```python
from build123d import *

# Parameters (mm, degrees)
SKETCH2_R           = 1.55
SKETCH2_R_2         = 6
SKETCH2_R_3         = 2.5
BOSS_EXTRUDE1_DEPTH = 3.2


with BuildPart() as part:
    # Sketch2 → Boss-Extrude1 (new body)
    with BuildSketch(Plane.XY):
        with BuildLine():
            Line((-37.606688888, -62.799107474), (37.606688888, -62.799107474))
            ThreePointArc((37.606688888, -62.799107474), (48.801571995, -62.445486831), (59.972328875, -61.630228563))
            ThreePointArc((59.972328875, -61.630228563), (73.015089975, -59.821162533), (85.558909279, -55.816298707))
            ThreePointArc((85.558909279, -55.816298707), (91.976349194, -50.332295109), (93.972328875, -42.130228563))
            Line((93.972328875, -42.130228563), (93.027953895, -29.351478281))
            ThreePointArc((93.027953895, -29.351478281), (95.742249073, -22.868177437), (101.827930469, -19.351777277))
            ThreePointArc((101.827930469, -19.351777277), (109.903770401, -18.491114916), (118, -19.132205072))
            ThreePointArc((118, -19.132205072), (125.861366739, -23.634125523), (129, -32.132205072))
            ThreePointArc((129, -32.132205072), (127.471762842, -56.297585918), (122.65808311, -80.027938374))
            ThreePointArc((122.65808311, -80.027938374), (122.741653332, -82.9548656), (124.449843954, -85.333094304))
            ThreePointArc((124.449843954, -85.333094304), (134.106812923, -89.628818458), (144.665008336, -89.144251365))
            ThreePointArc((144.665008336, -89.144251365), (146.218821849, -87.253980838), (145, -85.132205072))
            ThreePointArc((145, -85.132205072), (156.646327108, -43.296671083), (159.999998592, 0))
            ThreePointArc((159.999998592, 0), (152.263680347, 39.087893918), (134.999998592, 75))
            ThreePointArc((134.999998592, 75), (122.785714167, 86.318698338), (107.103701402, 91.920140268))
            ThreePointArc((107.103701402, 91.920140268), (53.654087158, 86.806881933), (0, 84.746395368))
            ThreePointArc((0, 84.746395368), (-53.654087158, 86.806881933), (-107.103701402, 91.920140268))
            ThreePointArc((-107.103701402, 91.920140268), (-122.785714167, 86.318698338), (-134.999998592, 75))
            ThreePointArc((-134.999998592, 75), (-152.263680347, 39.087893918), (-159.999998592, 0))
            ThreePointArc((-159.999998592, 0), (-156.646327108, -43.296671083), (-145, -85.132205072))
            ThreePointArc((-145, -85.132205072), (-146.218821849, -87.253980838), (-144.665008336, -89.144251365))
            ThreePointArc((-144.665008336, -89.144251365), (-134.106812923, -89.628818458), (-124.449843954, -85.333094304))
            ThreePointArc((-124.449843954, -85.333094304), (-122.741653332, -82.9548656), (-122.65808311, -80.027938374))
            ThreePointArc((-122.65808311, -80.027938374), (-127.471762842, -56.297585918), (-129, -32.132205072))
            ThreePointArc((-129, -32.132205072), (-125.861366739, -23.634125523), (-118, -19.132205072))
            ThreePointArc((-118, -19.132205072), (-109.903770401, -18.491114916), (-101.827930469, -19.351777277))
            ThreePointArc((-101.827930469, -19.351777277), (-95.742249073, -22.868177437), (-93.027953895, -29.351478281))
            Line((-93.027953895, -29.351478281), (-93.972328875, -42.130228563))
            ThreePointArc((-93.972328875, -42.130228563), (-91.976349194, -50.332295109), (-85.558909279, -55.816298707))
            ThreePointArc((-85.558909279, -55.816298707), (-73.015089975, -59.821162533), (-59.972328875, -61.630228563))
            ThreePointArc((-59.972328875, -61.630228563), (-48.801571995, -62.445486831), (-37.606688888, -62.799107474))
        make_face()
        with Locations((145.027741118, -2.999996549)):
            Circle(SKETCH2_R, mode=Mode.SUBTRACT)
        with Locations((80.027671125, 20)):
            Circle(SKETCH2_R_2, mode=Mode.SUBTRACT)
        with Locations((140.027625835, -59.000005176)):
            Circle(SKETCH2_R, mode=Mode.SUBTRACT)
        with Locations((129.987526969, 46.510623474)):
            Circle(SKETCH2_R_2, mode=Mode.SUBTRACT)
        with Locations((65.027671125, 5)):
            Circle(SKETCH2_R_2, mode=Mode.SUBTRACT)
        with Locations((0, 35)):
            Circle(SKETCH2_R_3, mode=Mode.SUBTRACT)
        with Locations((30.310889132, 17.5)):
            Circle(SKETCH2_R_3, mode=Mode.SUBTRACT)
        with Locations((30.310889132, -17.5)):
            Circle(SKETCH2_R_3, mode=Mode.SUBTRACT)
        with Locations((0, -35)):
            Circle(SKETCH2_R_3, mode=Mode.SUBTRACT)
        with Locations((-30.310889132, -17.5)):
            Circle(SKETCH2_R_3, mode=Mode.SUBTRACT)
        with Locations((-30.310889132, 17.5)):
            Circle(SKETCH2_R_3, mode=Mode.SUBTRACT)
        with Locations((-65.027671125, 5)):
            Circle(SKETCH2_R_2, mode=Mode.SUBTRACT)
        with Locations((-129.987526969, 46.510623474)):
            Circle(SKETCH2_R_2, mode=Mode.SUBTRACT)
        with Locations((-140.027625835, -59.000005176)):
            Circle(SKETCH2_R, mode=Mode.SUBTRACT)
        with Locations((-80.027671125, 20)):
            Circle(SKETCH2_R_2, mode=Mode.SUBTRACT)
        with Locations((-145.027741118, -2.999996549)):
            Circle(SKETCH2_R, mode=Mode.SUBTRACT)
        with BuildLine():
            Line((88.932649847, 20), (88.932649847, 38.765088603))
            ThreePointArc((88.932649847, 38.765088603), (93.755318616, 47.8620051), (103.122117375, 52.136944261))
            ThreePointArc((103.122117375, 52.136944261), (109.007507929, 50.935597689), (113.169909334, 46.604839083))
            Line((113.169909334, 46.604839083), (119.972328875, 33))
            ThreePointArc((119.972328875, 33), (121.177690194, 28.070536132), (120.972328875, 23))
            ThreePointArc((120.972328875, 23), (112.239255936, 12.094273751), (98.596517329, 9.081449277))
            ThreePointArc((98.596517329, 9.081449277), (91.695615864, 12.709508168), (88.932649847, 20))
        make_face(mode=Mode.SUBTRACT)
        with BuildLine():
            Line((-113.169909334, 46.604839083), (-119.972328875, 33))
            ThreePointArc((-119.972328875, 33), (-121.177690194, 28.070536132), (-120.972328875, 23))
            ThreePointArc((-120.972328875, 23), (-112.239255936, 12.094273751), (-98.596517329, 9.081449277))
            ThreePointArc((-98.596517329, 9.081449277), (-91.695615864, 12.709508168), (-88.932649847, 20))
            Line((-88.932649847, 20), (-88.932649847, 38.765088603))
            ThreePointArc((-88.932649847, 38.765088603), (-93.755318616, 47.8620051), (-103.122117375, 52.136944261))
            ThreePointArc((-103.122117375, 52.136944261), (-109.007507929, 50.935597689), (-113.169909334, 46.604839083))
        make_face(mode=Mode.SUBTRACT)
    extrude(amount=BOSS_EXTRUDE1_DEPTH)


solid = part.part
```
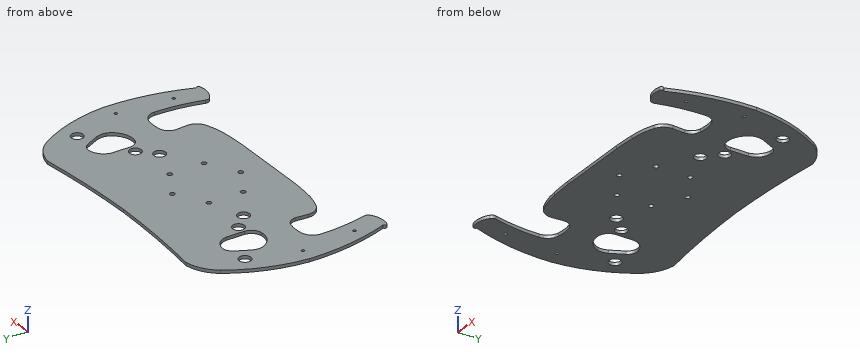
Read the model definition and answer for the solid it produces. Units are mm, in the model's axes. Round coordinates to 2 decimals unless told otherwise and drop trailing zeros. Write each loop counter-clockwise with the first axis right and the second up, starting at its lowest first coordinate (ties: lowest second). Pieces come first, ordered by that corner, then holes. Notation, with made-up numbers: (-33.5, 47) -> (18.5, 47) arc R7 cw to (18.5, 56) -> close; hole circle Ø1 at (76, 70.5). An arc over 180 degrees is marked (long way). Answer in a Markdown table with one row per item. Add a question column.
1) Find section D-D, the plane y = 58. Determine the outline of the cut face in (x, z), and give its area (3 significant figures).
2) Find section A-A, the plane y = -77. Determine the outline of the cut face in (x, z).
3) Find section C-C, the plane z = 2.6. State how many separate pieces and enclosed holes the cut face has, and give its area (3 significant figures).
4) Given P1, Ø2.5, axis at x = -145.03, y = -3, coming from the +Z side; P2, Ø1.6, axis at y = 31, z = 2, coming from the -X side, each flat-ended and moving along its own axis, determine where each tip first touches the part or whether it passes through.
5) Find section B-B, the plane y = 5. Determine the outline of the cut face in (x, z), and give its area (3 significant figures).
6) Consider line 1 (X direction, y = 6, z = 2.7); line 2 (X direction, y = -41.5, z = 0.2); line 3 (X direction, y = 47.5, z = 1.1). Determine where each line is inside the solid, lowest interval first.
Findings below:
| question | item | result |
|---|---|---|
| 1 | outline | (-144.57, 0) -> (144.57, 0) -> (144.57, 3.2) -> (-144.57, 3.2) -> close |
| 1 | area | 925 mm² |
| 2 | outline | (-147.96, 0) -> (-123.46, 0) -> (-123.46, 3.2) -> (-147.96, 3.2) -> close; (123.46, 0) -> (147.96, 0) -> (147.96, 3.2) -> (123.46, 3.2) -> close |
| 3 | separate pieces | 1 |
| 3 | enclosed holes | 18 |
| 3 | area | 40,600 mm² |
| 4 | P1 | through |
| 4 | P2 | x = -154.94 |
| 5 | outline | (-159.57, 0) -> (-71.03, 0) -> (-71.03, 3.2) -> (-159.57, 3.2) -> close; (-59.03, 0) -> (59.03, 0) -> (59.03, 3.2) -> (-59.03, 3.2) -> close; (71.03, 0) -> (159.57, 0) -> (159.57, 3.2) -> (71.03, 3.2) -> close |
| 5 | area | 944 mm² |
| 6 | line 1 | -159.47 to -70.94, -59.11 to 59.11, 70.94 to 159.47 |
| 6 | line 2 | -156.96 to -128.8, -93.93 to 93.93, 128.8 to 156.96 |
| 6 | line 3 | -149.19 to -135.91, -124.07 to -112.66, -93.38 to 93.38, 112.66 to 124.07, 135.91 to 149.19 |
